The model under review builds one solid part; all positions refer to its coordinate system, in mm. A direction names the side the tool comes from. Round coordinates to 2 decimals unless told otherwise and drop trailing zeros. Order: outer loops, then holes, each group sorted by start corner. A loop starts at its lowest first (then second) coordinate and runs counter-clockwise, first axis right, second up. Notation, with made-up numbers: M -36,-11.5 L 19,-11.5 A19 cw 19,15.5 Z; hole C -10.75,63.25 d3. An arc over 180 degrees is marked long. Use a Markdown table: item, result. Add a question column.
1. The part is to be moulded in two halves that separate along X. For faces 5 (the flat face through (-11.134, 6.92, 2.44)), 6 (the flat face through (-4.07, 9.76, 2.44)), 7 (the flat face through (0, 0, 2)), say which applies: +X half, -X half, draft (parallel to the pull), parting line (faces both ways), or undercut.
2. Consider section C-C on y = 8. State the section outline as (x, z) points.
3. Consider section A-A on y = 10. State the section outline as (x, z) points (3 decimals), then the cut area to 3 significant figures.
4. Consider section B-B on x = -5. State the section outline as (y, z) points.
5. For faces 1 (the flat face through (8, 11.8, 2)), 2 (the flat face through (-13, 1.5, 2)), 3 (the flat face through (4.16, 9.86, 2.44)), 4 (the flat face through (-10.5, 12, 2)), list the 3-axis set-ups (+Z, -Z, +X, -X, +Y, -Y) from which the entire face can be reached by the end or side of a thin tool; tool diameter is ignored.
6. To check wall thickness, follow probe 1 along X at (y, z) = (6.75, 3.4); probe 2 along X at (y, z) = (7.75, 3.6); probe 3 along X at (y, z) = (1.75, 4.75). State the ranges of each line that lie inside material, in increasing order.
7. Consider section D-D on x = 1.5. State the section outline as (y, z) points, then the cut area to 3 significant figures.
8. Insertion check: P1, Ø1.2, axis at y = 3.5, z = 3, coming from the +X side; P2, Ø2, axis at x = -2.5, y = 11.5, coming from the +Z side; P3, Ø0.5, axis at y = 11.5, z = 2.5, coming from the +X side; P4, Ø0.5, axis at y = 12, z = 3, coming from the -X side. Each pin has a flat end and moves straight along its axis. Give the tip position at first contact, or say it passes through.
from build123d import *

# Parameters (mm, degrees)
F1_DEPTH = 4.95
F2_R     = 1


with BuildPart() as f1:
    # F0 (on Top) → F1 (new body)
    with BuildSketch(Plane.XY):
        Polygon((-16.25, 0), (0, 0), (16.25, 0), (16.25, 1.5), (10.5, 1.5), (10.5, 5.5), (11.75, 8.3), (12.75, 8.3), (10.5, 11.3), (10.5, 13.6000004441), (7.4805053882, 13.6000004441), (0, 5.1791056932), (-7.4805053882, 13.6000004441), (-10.5, 13.6000004441), (-10.5, 11.3), (-12.75, 8.3), (-11.75, 8.3), (-10.5, 5.5), (-10.5, 1.5), (-16.25, 1.5), align=None)
        Polygon((-10.2784717774, 8.9287042967), (-8.9, 10.7666666667), (-8.9, 11.8000004441), (-7.5543964098, 11.8000004441), (0, 4.1791056932), (7.5543964098, 11.8000004441), (8.9, 11.8000004441), (8.9, 10.7666666667), (10.2784717774, 8.9287042967), (8.9, 5.8409275153), (8.9, 2.5), (0, 2.5), (-8.9, 2.5), (-8.9, 5.8409275153), align=None, mode=Mode.SUBTRACT)
    extrude(amount=F1_DEPTH)

    # F2
    f2_edges = [f1.edges().sort_by_distance(p)[0] for p in [
        (-16.25, 0.75, 4.95),
        (-16.25, 0.75, 0),
        (16.25, 0.75, 4.95),
        (16.25, 0.75, 0),
        (-16.25, 0, 2.475),
        (16.25, 0, 2.475),
        (0, 5.179106, 2.475),
        (0, 4.179106, 2.475),
        (-10.5, 11.3, 2.475),
        (-10.5, 13.6, 2.475),
        (10.5, 13.6, 2.475),
        (10.5, 11.3, 2.475),
    ]]
    fillet(f2_edges, radius=F2_R)


solid = f1.part
Answer block:
| question | item | result |
|---|---|---|
| 1 | face 5 | -X half |
| 1 | face 6 | undercut |
| 1 | face 7 | draft |
| 2 | outline | M -11.62,0 L -9.86,0 L -9.86,4.95 L -11.62,4.95 Z; M -3.79,0 L -2.51,0 L -2.51,4.95 L -3.79,4.95 Z; M 2.51,0 L 3.79,0 L 3.79,4.95 L 2.51,4.95 Z; M 9.86,0 L 11.62,0 L 11.62,4.95 L 9.86,4.95 Z |
| 3 | outline | M -11.475,0 L -9.475,0 L -9.475,4.95 L -11.475,4.95 Z; M -5.77,0 L -4.283,0 L -4.283,4.95 L -5.77,4.95 Z; M 4.283,0 L 5.77,0 L 5.77,4.95 L 4.283,4.95 Z; M 9.475,0 L 11.475,0 L 11.475,4.95 L 9.475,4.95 Z |
| 3 | area | 34.5 mm^2 |
| 4 | outline | M 0,0 L 2.5,0 L 2.5,4.95 L 0,4.95 Z; M 9.22,0 L 10.81,0 L 10.81,4.95 L 9.22,4.95 Z |
| 5 | face 1 | +Z, -Z |
| 5 | face 2 | +Z, -Z, -X |
| 5 | face 3 | +Z, -Z, +Y |
| 5 | face 4 | +Z, -Z, -X, +Y |
| 6 | probe 1 | -11.06 to -9.31, -2.55 to -1.4, 1.4 to 2.55, 9.31 to 11.06 |
| 6 | probe 2 | -11.5 to -9.75, -3.54 to -2.28, 2.28 to 3.54, 9.75 to 11.5 |
| 6 | probe 3 | -10.5 to 10.5 |
| 7 | outline | M 0,0 L 2.5,0 L 2.5,4.95 L 0,4.95 Z; M 5.69,0 L 6.87,0 L 6.87,4.95 L 5.69,4.95 Z |
| 7 | area | 18.2 mm^2 |
| 8 | P1 | x = 10.5 |
| 8 | P2 | through |
| 8 | P3 | x = 10.58 |
| 8 | P4 | x = -10.5 |
